from build123d import *

# Parameters (mm, degrees)
F0_R     = 9
F1_DEPTH = 5


with BuildPart() as f1:
    # F0 (on Top) → F1 (new body)
    with BuildSketch(Plane.XY):
        with BuildLine():
            ThreePointArc((-19.295465, 13.710922), (-8.5, 14.722432), (-2.226274, 23.565824))
            ThreePointArc((-2.226274, 23.565824), (-2.056692, 24.768004), (-2, 25.980762))
            ThreePointArc((-2, 25.980762), (-22.521933, 36.583617), (-19.295465, 13.710922))
        make_face()
        with Locations((-15, 25.980762)):
            Circle(F0_R, mode=Mode.SUBTRACT)
        with BuildLine():
            ThreePointArc((8.478261, -9.854902), (11.815612, -5.421375), (13, 0))
            ThreePointArc((13, 0), (11.815612, 5.421375), (8.478261, 9.854902))
            ThreePointArc((8.478261, 9.854902), (6.5, 11.25833), (4.295465, 12.26984))
            ThreePointArc((4.295465, 12.26984), (-6.5, 11.25833), (-12.773726, 2.414938))
            ThreePointArc((-12.773726, 2.414938), (-13, 0), (-12.773726, -2.414938))
            ThreePointArc((-12.773726, -2.414938), (-6.5, -11.25833), (4.295465, -12.26984))
            ThreePointArc((4.295465, -12.26984), (6.5, -11.25833), (8.478261, -9.854902))
        make_face()
        Circle(F0_R, mode=Mode.SUBTRACT)
        with BuildLine():
            ThreePointArc((-12.773726, 2.414938), (-6.5, 11.25833), (4.295465, 12.26984))
            ThreePointArc((4.295465, 12.26984), (-1.060585, 16.708179), (-2.226274, 23.565824))
            ThreePointArc((-2.226274, 23.565824), (-8.5, 14.722432), (-19.295465, 13.710922))
            ThreePointArc((-19.295465, 13.710922), (-13.939415, 9.272583), (-12.773726, 2.414938))
        make_face()
        with BuildLine():
            ThreePointArc((8.478261, 9.854902), (11.815612, 5.421375), (13, 0))
            ThreePointArc((13, 0), (11.815612, -5.421375), (8.478261, -9.854902))
            ThreePointArc((8.478261, -9.854902), (15, -7.435596), (21.521739, -9.854902))
            ThreePointArc((21.521739, -9.854902), (17, 0), (21.521739, 9.854902))
            ThreePointArc((21.521739, 9.854902), (15, 7.435596), (8.478261, 9.854902))
        make_face()
        with BuildLine():
            ThreePointArc((43, 0), (35.421375, 11.815612), (21.521739, 9.854902))
            ThreePointArc((21.521739, 9.854902), (17, 0), (21.521739, -9.854902))
            ThreePointArc((21.521739, -9.854902), (35.421375, -11.815612), (43, 0))
        make_face()
        with Locations((30, 0)):
            Circle(F0_R, mode=Mode.SUBTRACT)
        with BuildLine():
            ThreePointArc((-2.226274, -23.565824), (-1.060585, -16.708179), (4.295465, -12.26984))
            ThreePointArc((4.295465, -12.26984), (-6.5, -11.25833), (-12.773726, -2.414938))
            ThreePointArc((-12.773726, -2.414938), (-13.939415, -9.272583), (-19.295465, -13.710922))
            ThreePointArc((-19.295465, -13.710922), (-8.5, -14.722432), (-2.226274, -23.565824))
        make_face()
        with BuildLine():
            ThreePointArc((-2, -25.980762), (-2.056692, -24.768004), (-2.226274, -23.565824))
            ThreePointArc((-2.226274, -23.565824), (-8.5, -14.722432), (-19.295465, -13.710922))
            ThreePointArc((-19.295465, -13.710922), (-22.521933, -36.583617), (-2, -25.980762))
        make_face()
        with Locations((-15, -25.980762)):
            Circle(F0_R, mode=Mode.SUBTRACT)
    extrude(amount=F1_DEPTH)


solid = f1.part
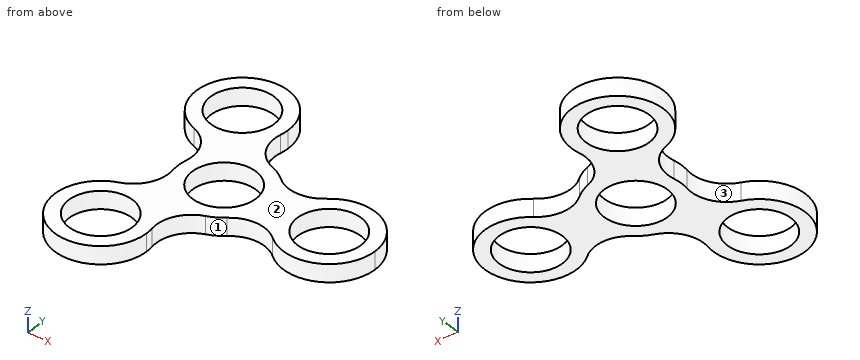
Read the model definition and answer for the solid it produces. Units are mm, in the model's axes. Face numbers are marked on the shaded views. Give positions to 0.01 mm unless a question says otherwise; leave off trailing zeros. Write each loop counter-clockwise with the first axis right and the second up, starting at its lowest first coordinate (ties: lowest second). Pieces come first, ordered by that corner, then holes. Notation, with made-up numbers: (15.25, 80) -> (39.25, 80) arc R19 ccw to (39.25, 88) -> close; hole circle Ø8 at (-6.5, 81). An arc over 180 degrees is marked (long way). Answer as a JSON object with one key per item and string values. Group by question number.
1) Find section A-A (x = 30). Write down the section's boundary in (y, z), and give its area (3 significant figures).
2) The mould has two halves that part along X. Classify the marked faces 1, 2 and 3: +X half, -X half, draft (parallel to the pull), parting line (faces both ways), or undercut.
3) Each of these flat-tipped pins is pushed along its axis until it touches: P1, Ø1, axis at x = 23, z = 4.5, coming from the +Y side; P2, Ø1.5, axis at x = 12, z = 1, coming from the +Y side; P3, Ø11, axis at x = 30, y = 0, coming from the +Z side; P4, Ø1, axis at y = -20.5, z = 3.5, coming from the -X side. Where does it stop, or does it pass through?
4) Find section B-B (z = 3.35). Write down the section's boundary in (x, y).
5) Find section D-D (x = -23). Write down the section's boundary in (y, z), and give its area (3 significant figures).
6) Find section C-C (y = 34). Write down the section's boundary in (x, z).
7) Consider L1, parallel to X at y = -7, z = 2.9; L2, parallel to Y at x = -17.5, z = 2.9; L3, parallel to Y at x = -21.5, z = 2.4. Determine where each line is inside the solid, lowest interval first. Write a range as from..to.
Values follow:
{
 "1": {"outline": "(-13, 0) -> (-9, 0) -> (-9, 5) -> (-13, 5) -> close; (9, 0) -> (13, 0) -> (13, 5) -> (9, 5) -> close", "area": "40.0 mm2"},
 "2": {"face 1": "undercut", "face 2": "draft", "face 3": "-X half"},
 "3": {"P1": "stops at y = 11.26", "P2": "stops at y = 8.17", "P3": "passes through", "P4": "stops at x = -27.01"},
 "4": {"outline": "(-19.3, -13.71) arc R13 ccw (long way) to (-2, -25.98) arc R13 ccw to (-2.23, -23.57) arc R10 cw to (4.3, -12.27) arc R13 ccw to (8.48, -9.85) arc R10 cw to (21.52, -9.85) arc R13 ccw (long way) to (21.52, 9.85) arc R10 cw to (8.48, 9.85) arc R13 ccw to (4.3, 12.27) arc R10 cw to (-2.23, 23.57) arc R13 ccw to (-2, 25.98) arc R13 ccw (long way) to (-19.3, 13.71) arc R10 cw to (-12.77, 2.41) arc R13 ccw to (-12.77, -2.41) arc R10 cw to start; hole circle Ø18 at (-15, -25.98); hole circle Ø18 at (-15, 25.98); hole circle Ø18 at (0, 0); hole circle Ø18 at (30, 0)"},
 "5": {"outline": "(-36.23, 0) -> (-30.1, 0) -> (-30.1, 5) -> (-36.23, 5) -> close; (-21.86, 0) -> (-15.73, 0) -> (-15.73, 5) -> (-21.86, 5) -> close; (15.73, 0) -> (21.86, 0) -> (21.86, 5) -> (15.73, 5) -> close; (30.1, 0) -> (36.23, 0) -> (36.23, 5) -> (30.1, 5) -> close", "area": "122 mm2"},
 "6": {"outline": "(-25.23, 0) -> (-19.09, 0) -> (-19.09, 5) -> (-25.23, 5) -> close; (-10.91, 0) -> (-4.77, 0) -> (-4.77, 5) -> (-10.91, 5) -> close"},
 "7": {"L1": "x = -12.98..-5.66, 5.66..24.34, 35.66..40.95", "L2": "y = -38.74..-34.63, -17.33..-12.87, 12.87..17.33, 34.63..38.74", "L3": "y = -37.24..-32.21, -19.76..-14.72, 14.72..19.76, 32.21..37.24"}
}
